```python
from build123d import *

# Parameters (mm, degrees)
SKETCH1_R              = 14.2875
BOSS_EXTRUDE1_DEPTH    = 12.7
SKETCH2_R              = 2.413
INITIAL_MOUNTING_DEPTH = 13.7
MOUNTING_PATTERN_COUNT = 8
FILLET1_R              = 6.35
SKETCH3_R              = 2.413
CUT_EXTRUDE1_DEPTH     = 26.4
CUT_EXTRUDE2_START     = -12.7
SKETCH3_3_R            = 4.445
SKETCH3_3_R_2          = 2.413
CUT_EXTRUDE2_DEPTH     = 13.7
SKETCH4_R              = 2.413
CUT_EXTRUDE3_DEPTH     = 13.7
LPATTERN1_COUNT        = 5
LPATTERN1_PITCH        = 12.7
CUT_EXTRUDE4_START     = -12.7
SKETCH5_R              = 4.445
CUT_EXTRUDE4_DEPTH     = 6.35
CIRPATTERN1_COUNT      = 8


with BuildPart() as part:
    # Sketch1 → Boss-Extrude1 (new body)
    with BuildSketch(Plane.XY):
        Polygon((-63.5, -42.607736074), (63.5, -42.607736074), (50.06388407, 33.592263926), (-50.06388407, 33.592263926), (-88.9, 33.592263926), (-88.9, 8.192263926), (-63.5, 8.192263926), align=None)
        with Locations((-12.04252973, -7.815733859)):
            Circle(SKETCH1_R, mode=Mode.SUBTRACT)
    extrude(amount=BOSS_EXTRUDE1_DEPTH)

    # Sketch2 → Initial Mounting (cut, through all)
    with BuildSketch(Plane.XY.offset(12.7)):
        with Locations((-12.04252973, -33.215733859)):
            Circle(SKETCH2_R)
    initial_mounting = extrude(amount=-INITIAL_MOUNTING_DEPTH, mode=Mode.SUBTRACT)

    # Mounting Pattern: Initial Mounting ×8 about axis
    mounting_pattern_axis = Axis((-12.04252973, -7.815733859, 0), (0, 0, 1))
    for i in range(1, MOUNTING_PATTERN_COUNT):
        add(initial_mounting.rotate(mounting_pattern_axis, i * 360 / MOUNTING_PATTERN_COUNT), mode=Mode.SUBTRACT)

    # Fillet1
    fillet1_edges = [part.edges().sort_by_distance(p)[0] for p in [
        (63.5, -42.607736074, 6.35),
        (-63.5, -42.607736074, 6.35),
        (-88.9, 33.592263926, 6.35),
        (50.06388407, 33.592263926, 6.35),
    ]]
    fillet(fillet1_edges, radius=FILLET1_R)

    # Sketch3 → Cut-Extrude1 (cut, through all)
    with BuildSketch(Plane.XZ.offset(-8.192263926)):
        with Locations((-76.327, 6.35)):
            Circle(SKETCH3_R)
    extrude(amount=-CUT_EXTRUDE1_DEPTH, mode=Mode.SUBTRACT)

    # Sketch3<3> → Cut-Extrude2 (cut, through all)
    with BuildSketch(Plane.XZ.offset(-8.192263926).offset(CUT_EXTRUDE2_START)):
        with Locations((-76.327, 6.35)):
            Circle(SKETCH3_3_R)
        with Locations((-76.327, 6.35)):
            Circle(SKETCH3_3_R_2, mode=Mode.SUBTRACT)
    extrude(amount=-CUT_EXTRUDE2_DEPTH, mode=Mode.SUBTRACT)

    # Sketch4 → Cut-Extrude3 (cut, through all)
    with BuildSketch(Plane.XY.offset(12.7)):
        with Locations((48.364729374, -29.907736074)):
            Circle(SKETCH4_R)
    cut_extrude3 = extrude(amount=-CUT_EXTRUDE3_DEPTH, mode=Mode.SUBTRACT)

    # LPattern1: Cut-Extrude3 ×5
    with Locations(*[Vector(-0.173648178, 0.984807753, 0) * (i * LPATTERN1_PITCH) for i in range(1, LPATTERN1_COUNT)]):
        add(cut_extrude3, mode=Mode.SUBTRACT)

    # Sketch5 → Cut-Extrude4 (cut)
    with BuildSketch(Plane(origin=(0, 0, 0), x_dir=(-1, 0, 0), z_dir=(0, 0, -1)).offset(CUT_EXTRUDE4_START)):
        with Locations((12.04252973, 17.584266141)):
            Circle(SKETCH5_R)
    cut_extrude4 = extrude(amount=CUT_EXTRUDE4_DEPTH, mode=Mode.SUBTRACT)

    # CirPattern1: Cut-Extrude4 ×8 about axis
    cirpattern1_axis = Axis((-12.04252973, -7.815733859, 0), (0, 0, 1))
    for i in range(1, CIRPATTERN1_COUNT):
        add(cut_extrude4.rotate(cirpattern1_axis, i * 360 / CIRPATTERN1_COUNT), mode=Mode.SUBTRACT)


solid = part.part
```
Check sheet for the modelled part. Datum: model origin and axes. Units: mm. A direction names the side the tool comes from. Give positions to 0.01 mm unless a question says otherwise; leave off trailing zeros. Order: outer loops, then holes, each group sorted by start corner. A loop starts at its lowest first (then second) coordinate and runs counter-clockwise, first axis right, second up. Notation, with made-up numbers: M -19,-2.75 L -10,-2.75 A13 cw -10,22.25 Z; hole C 69.5,4.25 d3. An arc over 180 degrees is marked long. Answer in a Markdown table with one row per item. Add a question column.
Q1. Access from +Z, -Z, +X, -X, +Y, -Y to the whole of each face (thin tool, end or side, straight path). Record for faces 4 (the flat face through (-10, -31, 6.35)), 5 (the cylindrical face through (-35.05, -7.5, 3.22)).
Q2. Thickness scan on L1, parallel to X at y = -3.5, z = 1.5; L2, parallel to X at y = -8.5, z = 11.25; L3, parallel to X at y = -30.5, z = 12. Record the ranges inside material, lowest first.
Q3. Sectioned sample at A-A, the plane x = -76.5. Record the boundary of the cut face in (y, z), and give its area (3 significant figures).
Q4. Sectioned sample at B-B, the plane x = 52.5. Record the boundary of the cut face in (y, z).
Q5. Gauge pin test, flat ends, axial feed: pin 1 Ø7.5 at (x, y) = (5.92, 10.14) entering from +Z; pin 2 Ø8 at (x, y) = (-16.5, -24.5) entering from -Z; pin 3 Ø1.5 at (y, z) = (15, 7.5) entering from +X; pin 4 Ø7.5 at (x, z) = (-76.327, 6.35) entering from -Y. Record the tip position at first contact, or that the pin passes through.
Q6. Release check for a two-part mould opening along Y. For faces 1 (the flat face through (-63.5, -14, 6)), 2 (the flat face through (-73.6, 8.192, 6.3)), 3 (the flat face through (6, -23, 6.35)) record: released by +Y, released by -Y, zero draft, split by the parting line, or undercut.
Verdict:
| question | item | result |
|---|---|---|
| 1 | face 4 | +Z |
| 1 | face 5 | +Z, -Z |
| 2 | L1 | -63.5 to -25.66, 1.58 to 41.98, 45.92 to 56.6 |
| 2 | L2 | -63.5 to -41.83, -33.05 to -26.31, 2.23 to 8.97, 17.75 to 57.49 |
| 2 | L3 | -63.5 to -15.56, -8.52 to 46.03, 50.7 to 61.37 |
| 3 | outline | M 8.19,0 L 33.59,0 L 33.59,1.91 L 20.89,1.91 L 20.89,3.94 L 8.19,3.94 Z; M 8.19,8.76 L 20.89,8.76 L 20.89,10.79 L 33.59,10.79 L 33.59,12.7 L 8.19,12.7 Z |
| 3 | area | 149 mm² |
| 4 | outline | M -42.61,0 L 19.78,0 L 19.78,12.7 L -42.61,12.7 Z |
| 5 | pin 1 | z = 6.35 |
| 5 | pin 2 | z = 0 |
| 5 | pin 3 | x = 53.47 |
| 5 | pin 4 | y = 8.19 |
| 6 | face 1 | zero draft |
| 6 | face 2 | released by -Y |
| 6 | face 3 | undercut |
